from build123d import *

# Parameters (mm, degrees)
BOSS_EXTRUDE1_DEPTH = 11.43
BOSS_EXTRUDE2_DEPTH = 77.866799282


with BuildPart() as part:
    # Sketch1 → Boss-Extrude1 (new body)
    with BuildSketch(Plane(origin=(0, 68.54, 0), x_dir=(1, 0, 0), z_dir=(0, 1, 0))):
        with BuildLine():
            Line((-505.199519379, -28.941561379), (-510.924193781, -42.454904444))
            Line((-510.924193781, -42.454904444), (-446.727083924, -108.742597242))
            Line((-446.727083924, -108.742597242), (-432.506297568, -99.706904201))
            Line((-432.506297568, -99.706904201), (-453.485090126, -44.423263798))
            ThreePointArc((-453.485090126, -44.423263798), (-468.76509838, -42.570216845), (-475.918740123, -28.941649602))
            Line((-475.918740123, -28.941649602), (-505.199519379, -28.941561379))
        make_face()
    extrude(amount=-BOSS_EXTRUDE1_DEPTH)

    # Sketch4 → Boss-Extrude2 (add)
    with BuildSketch(Plane(origin=(0, -20.756799282, 0), x_dir=(1, 0, 0), z_dir=(0, 1, 0))):
        Polygon((-505.199519379, -28.941561379), (-510.924193781, -42.454904444), (-475.918740123, -42.454904444), (-475.918740123, -28.941649602), align=None)
    extrude(amount=BOSS_EXTRUDE2_DEPTH)


solid = part.part
Check sheet for the modelled part. Datum: model origin and axes. Units: mm. A direction names the side the tool comes from. Give positions to 0.01 mm unless a question says otherwise; leave off trailing zeros. Order: outer loops, then holes, each group sorted by start corner. A loop starts at its lowest first (then second) coordinate and runs counter-clockwise, first axis right, second up. Notation, with made-up numbers: M -17,52 L 22,52 A16 ccw 22,74 Z; hole C 7,45 d7. An arc over 180 degrees is marked long. Answer as CSV lines item,"result". Start each with the question number.
Item 1: Thickness scan on line 1 (Y direction, x = -491.5, z = 46); line 2 (Z direction, x = -483.5, y = -10.5); line 3 (Z direction, x = -478, y = 62). Record the ranges inside material, lowest first. Write a range as [from, to].
Item 2: Cross-section at C-C on z = 87. Enter the section's corners in (x, y).
Item 3: Cross-section at B-B on y = 51. Enter the section's corners in (x, z), plus the area to 3 significant figures.
Item 4: Cross-section at A-A on x = -499. Enter the section's corners in (y, z), plus the area to 3 significant figures.
Item 5: Gauge pin test, flat ends, axial feed: P1, Ø3, axis at x = -493.5, z = 64, coming from the +Y side; P2, Ø17.5, axis at x = -499.5, y = 3.5, coming from the +Z side; P3, Ø15, axis at y = 37.5, z = 36.5, coming from the +X side; P4, Ø23.5, axis at x = -461.5, z = 68.5, coming from the -Y side. Record the tip position at first contact, or that the pin passes through.
Item 6: Tool access check on faces 1 (the face through (-494, 18, 42.455)), 2 (the face through (-494, -20.757, 36)), 3 (the face through (-475.919, 18, 36)). Record the directions out of +Z, -Z, +X, -X, +Y, -Y that give a thin tool (end or side, any length) a straight path to the whole face; none if there is none.
Established:
1,line 1,"y = [57.11, 68.54]"
1,line 2,"z = [28.94, 42.45]"
1,line 3,"z = [28.94, 76.45]"
2,outline,"M -467.78,57.11 L -437.33,57.11 L -437.33,68.54 L -467.78,68.54 Z"
3,outline,"M -510.92,42.45 L -505.2,28.94 L -475.92,28.94 L -475.92,42.45 Z"
3,area,"434 mm^2"
4,outline,"M -20.76,28.94 L 68.54,28.94 L 68.54,54.77 L 57.11,54.77 L 57.11,42.45 L -20.76,42.45 Z"
4,area,"1,350 mm^2"
5,P1,"passes through"
5,P2,"stops at z = 42.45"
5,P3,"stops at x = -475.92"
5,P4,"stops at y = 57.11"
6,face 1,"+Z, +X, -X, -Y"
6,face 2,"+Z, -Z, +X, -X, -Y"
6,face 3,"+Z, -Z, +X, -Y"
